```python
from build123d import *

# Parameters (mm, degrees)
SKETCH_1_R      = 2.5
EXTRUDE_1_DEPTH = 170
FILLET_1_R      = 1.5
FILLET_2_R      = 0.2


with BuildPart() as part:
    # 草图1 → 凸台-拉伸1 (new body)
    with BuildSketch(Plane.XY):
        Polygon((-9.999999566, 9.999999566), (-4.399999566, 9.999999566), (-4.399999566, 9.499999566), (-3.899999566, 9.499999566), (-3.899999566, 8.199999566), (-5.899999566, 8.199999566), (-5.899999566, 6.960659737), (-2.839609534, 3.900132646), (2.839471605, 3.900132646), (5.900000434, 6.960661475), (5.900000434, 8.200001303), (3.900000434, 8.200001303), (3.900000434, 9.500001303), (4.400000434, 9.500001303), (4.400000434, 10.000001303), (10.000000434, 10.000001303), (10.000000434, 4.400001303), (9.500000434, 4.400001303), (9.500000434, 3.900001303), (8.200000434, 3.900001303), (8.200000434, 5.900001303), (6.960660606, 5.900001303), (3.900133515, 2.839611272), (3.900133515, -2.839469868), (6.960662344, -5.899998697), (8.200002172, -5.899998697), (8.200002172, -3.899998697), (9.500002172, -3.899998697), (9.500002172, -4.399998697), (10.000002172, -4.399998697), (10.000000434, -10.000000434), (4.400002172, -9.999998697), (4.400002172, -9.499998697), (3.900002172, -9.499998697), (3.900002172, -8.199998697), (5.900002172, -8.199998697), (5.900002172, -6.960658869), (2.839475081, -3.899994711), (-2.839331933, -3.899994711), (-5.899997828, -6.960660606), (-5.899997828, -8.200000434), (-3.899997828, -8.200000434), (-3.899997828, -9.500000434), (-4.399997828, -9.500000434), (-4.399997828, -10.000000434), (-9.999999566, -10.000000434), (-9.999997828, -4.400000434), (-9.499997828, -4.400000434), (-9.499997828, -3.900000434), (-8.199997828, -3.900000434), (-8.199997828, -5.900000434), (-6.960658, -5.900000434), (-3.899993842, -2.839473343), (-3.899993842, 2.83933367), (-6.960659737, 5.899999566), (-8.199999566, 5.899999566), (-8.199999566, 3.899999566), (-9.499999566, 3.899999566), (-9.499999566, 4.399999566), (-9.999999566, 4.399999566), align=None)
        Circle(SKETCH_1_R, mode=Mode.SUBTRACT)
    extrude(amount=EXTRUDE_1_DEPTH)

    # 圆角1
    fillet_1_edges = [part.edges().sort_by_distance(p)[0] for p in [
        (10.000000434, 10.000001303, 85),
        (10.000000434, -10.000000434, 85),
        (-9.999999566, -10.000000434, 85),
        (-9.999999566, 9.999999566, 85),
    ]]
    fillet(fillet_1_edges, radius=FILLET_1_R)

    # 圆角2
    fillet_2_edges = [part.edges().sort_by_distance(p)[0] for p in [
        (3.900133515, 2.839611272, 85),
        (3.900133515, -2.839469868, 85),
        (2.839475081, -3.899994711, 85),
        (-2.839331933, -3.899994711, 85),
        (-3.899993842, -2.839473343, 85),
        (-3.899993842, 2.83933367, 85),
        (-2.839609534, 3.900132646, 85),
        (2.839471605, 3.900132646, 85),
    ]]
    fillet(fillet_2_edges, radius=FILLET_2_R)


solid = part.part
```
Could you check a few things on this model? Use its own coordinates, in mm. A direction names the side the tool comes from. Give positions to 0.01 mm unless a question says otherwise; leave off trailing zeros. Loops run counter-clockwise (first coordinate to the right, second up) from the corner with the lowest first, then second, coordinate; pieces in that order, holes last. Notation, with made-up numbers: (-33.5, 57) -> (-10.5, 57) arc R10 ccw to (-10.5, 64) -> close; hole circle Ø9 at (85, 25). An arc over 180 degrees is marked (long way). Put each result on its own line as item: value.
(1) Imagine slicing it at A-A on y = 0. Write out the boundary of the cut face in (x, z), plus the area to 3 significant figures.
Computed:
outline: (-3.9, 0) -> (-2.5, 0) -> (-2.5, 170) -> (-3.9, 170) -> close; (2.5, 0) -> (3.9, 0) -> (3.9, 170) -> (2.5, 170) -> close
area: 476 mm^2
(2) Thinking about a two-plate mould opening in X: for faces 1 (the face through (5.44, -4.38, 83.81)), 2 (the face through (-4.38, -5.44, 83.81)), 3 (the face through (3.9, 0, 84)), 4 (the face through (6, 10, 84)), which applies, pulls with the +X half, pulls with the -X half, needs draft (parallel to the pull), parting line crosses it, or undercut?
Computed:
face 1: undercut
face 2: undercut
face 3: pulls with the +X half
face 4: needs draft
(3) Please list where these lines run through material, in increasing order: probe 1 along Y at (x, z) = (0, 122); probe 2 along X at (y, z) = (-4.75, 23.5); probe 3 along Y at (x, z) = (-5.5, 136). Write a range as [from, to].
Computed:
probe 1: [-3.9, -2.5], [2.5, 3.9]
probe 2: [-10, -8.2], [-5.81, -3.69], [3.69, 5.81], [8.2, 10]
probe 3: [-10, -8.2], [-6.56, -4.44], [4.44, 6.56], [8.2, 10]
(4) For faces 5 (the face through (-6, 10, 84)), 6 (the face through (0, 3.9, 84)), 7 (the face through (-5.44, 4.38, 83.81)), 8 (the face through (0, -3.9, 84)), 9 (the face through (-10, 6, 84)), which set-ups out of +Z, -Z, +X, -X, +Y, -Y let a thin tool reach every point of the face, with its end or its side?
Computed:
face 5: +Z, -Z, +X, -X, +Y
face 6: +Z, -Z, +Y
face 7: +Z, -Z
face 8: +Z, -Z, -Y
face 9: +Z, -Z, -X, +Y, -Y
(5) I'm going to push flat-ended pins straight in: pin 1 Ø0.6 at (y, z) = (-4, 105) entering from -X; pin 2 Ø8 at (x, z) = (-3, 106.5) entering from +Y; pin 3 Ø0.6 at (y, z) = (9, 104.5) entering from -X; pin 4 Ø1 at (x, z) = (3.5, 47.5) entering from -Y. Where does each tip first touch, or does it pass through?
Computed:
pin 1: x = -9.5
pin 2: y = 10
pin 3: x = -9.99
pin 4: y = -9.5
